Verification items for the finished model (mm, model axes). Give positions to 0.01 mm unless a question says otherwise; leave off trailing zeros. Loops run counter-clockwise (first coordinate to the right, second up) from the corner with the lowest first, then second, coordinate; pieces in that order, holes last. Notation, with made-up numbers: (-31.5, -8) - (3.5, -8) arc R38 ccw to (3.5, 30) - close; hole circle Ø4 at (-26, -37). An arc over 180 degrees is marked (long way). One line per item, written item: value. Start each with the question number.
1. Sectioned sample at A-A (y = 19.05). Record the cut outline in (x, z).
2. Sectioned sample at B-B (x = 19.05). Record the cut outline in (y, z).
3. Sectioned sample at C-C (z = 3). Count the separate pieces of the cut face and the enclosed holes in it, plus the area to 3 significant figures.
4. Gauge pin test, flat ends, axial feed: pin 1 (1.5 mm diameter, centred on y = 10, z = 5.5, fed in from +X); pin 2 (1.5 mm diameter, centred on x = 38, z = 5, fed in from +Y). Record the tip position at first contact, or that the pin passes through.
5. Sectioned sample at D-D (x = 58). Record the cut outline in (y, z).
6. Mould release check, pull along X, two halves, no side actions. Record for faces 1 (the cylindrical face through (38.633, 0.724, 5.586)), 2 (the cylindrical face through (18.595, 22.513, 3.219)), 3 (the cylindrical face through (0.724, 19.317, 5.586)): pulls with the +X half, pulls with the -X half, needs draft (parallel to the pull), parting line crosses it, or undercut.
7. Scan lines: L1, parallel to X at y = 21, z = 1.75; L2, parallel to X at y = 16, z = 3; L3, parallel to Y at x = 19.05, z = 2.75. Record each from-to range of solid material in increasing order. Write a range as [from, to].
from build123d import *

# Parameters (mm, degrees)
SKETCH1_W           = 76.2
SKETCH1_H           = 38.1
BOSS_EXTRUDE1_DEPTH = 6.35
FILLET1_R           = 2.54
SKETCH2_R           = 3.4925
CUT_EXTRUDE1_DEPTH  = 6.35


with BuildPart() as part:
    # Sketch1 → Boss-Extrude1 (new body)
    with BuildSketch(Plane.XY):
        with Locations((38.1, 19.05)):
            Rectangle(SKETCH1_W, SKETCH1_H)
    extrude(amount=BOSS_EXTRUDE1_DEPTH)

    # Fillet1
    fillet1_edges = [part.edges().sort_by_distance(p)[0] for p in [
        (76.2, 19.05, 6.35),
        (38.1, 38.1, 6.35),
        (0, 19.05, 6.35),
        (38.1, 0, 6.35),
    ]]
    fillet(fillet1_edges, radius=FILLET1_R)

    # Sketch2 → Cut-Extrude1 (cut)
    with BuildSketch(Plane.XY.offset(6.35)):
        with Locations((19.05, 19.05)):
            Circle(SKETCH2_R)
        with Locations((57.15, 19.05)):
            Circle(SKETCH2_R)
    extrude(amount=-CUT_EXTRUDE1_DEPTH, mode=Mode.SUBTRACT)


solid = part.part
Results are:
1. outline: (0, 0) - (15.56, 0) - (15.56, 6.35) - (2.54, 6.35) arc R2.54 ccw to (0, 3.81) - close; (22.54, 0) - (53.66, 0) - (53.66, 6.35) - (22.54, 6.35) - close; (60.64, 0) - (76.2, 0) - (76.2, 3.81) arc R2.54 ccw to (73.66, 6.35) - (60.64, 6.35) - close
2. outline: (0, 0) - (15.56, 0) - (15.56, 6.35) - (2.54, 6.35) arc R2.54 ccw to (0, 3.81) - close; (22.54, 0) - (38.1, 0) - (38.1, 3.81) arc R2.54 ccw to (35.56, 6.35) - (22.54, 6.35) - close
3. separate pieces: 1
3. enclosed holes: 2
3. area: 2,830 mm^2
4. pin 1: stops at x = 76.02
4. pin 2: stops at y = 38.06
5. outline: (0, 0) - (15.66, 0) - (15.66, 6.35) - (2.54, 6.35) arc R2.54 ccw to (0, 3.81) - close; (22.44, 0) - (38.1, 0) - (38.1, 3.81) arc R2.54 ccw to (35.56, 6.35) - (22.44, 6.35) - close
6. face 1: needs draft
6. face 2: undercut
6. face 3: pulls with the -X half
7. L1: x = [0, 16.15], [21.95, 54.25], [60.05, 76.2]
7. L2: x = [0, 17.35], [20.75, 55.45], [58.85, 76.2]
7. L3: y = [0, 15.56], [22.54, 38.1]
